Design review of the part built by this model. Coordinates are the model's own, in mm. Coordinates: 2 decimals unless noted, no trailing zeros. Write each loop counter-clockwise with the first axis right and the second up, starting at its lowest first coordinate (ties: lowest second). Pieces come first, ordered by that corner, then holes. Notation, with made-up numbers: (-35.5, 42.25) - (-25.5, 42.25) arc R29 ccw to (-25.5, 71.25) - close; hole circle Ø10 at (-17, 35.5). An arc over 180 degrees is marked (long way). One line per item, written item: value.
from build123d import *

# Parameters (mm, degrees)
CYLINDER021_R       = 5
CYLINDER021_DEPTH   = 15
CYLINDER107_R       = 1.6
CYLINDER107_DEPTH   = 20
ARRAY001008_X_COUNT = 2
ARRAY001008_X_PITCH = 22
ARRAY001008_Y_COUNT = 2
ARRAY001008_Y_PITCH = 22
BOX009_W            = 30
BOX009_H            = 30
BOX009_DEPTH        = 1
FILLET004_R         = 4


with BuildPart() as side_bearing_central_hole_cylinder001:
    # Cylinder021 → Cylinder021 (new body)
    with BuildSketch(Plane(origin=(15, 15, -4), x_dir=(1, 0, 0), z_dir=(0, 0, 1))):
        Circle(CYLINDER021_R)
    extrude(amount=CYLINDER021_DEPTH)


with BuildPart() as fusion010:
    # Cylinder107 → Cylinder107 (new body)
    with BuildSketch(Plane(origin=(4, 4, -7), x_dir=(1, 0, 0), z_dir=(0, 0, 1))):
        Circle(CYLINDER107_R)
    extrude(amount=CYLINDER107_DEPTH)

    # Array001008 X: Fusion010 ×2


with BuildPart() as fusion010_1:
    add(fusion010.part)
    with Locations(*[(i * ARRAY001008_X_PITCH, 0, 0) for i in range(1, ARRAY001008_X_COUNT)]):
        add(fusion010.part)

    # Array001008 Y: Fusion010 ×2


with BuildPart() as fusion010_2:
    add(fusion010_1.part)
    with Locations(*[(0, i * ARRAY001008_Y_PITCH, 0) for i in range(1, ARRAY001008_Y_COUNT)]):
        add(fusion010_1.part)

    # Fusion010: union side bearing central hole cylinder001
    add(side_bearing_central_hole_cylinder001.part)


with BuildPart() as bearing_cover_fillet:
    # Box009 → Box009 (new body)
    with BuildSketch(Plane.XY):
        with Locations((15, 15)):
            Rectangle(BOX009_W, BOX009_H)
    extrude(amount=BOX009_DEPTH)

    # Cut007: cut Fusion010
    add(fusion010_2.part, mode=Mode.SUBTRACT)

    # Fillet004
    fillet004_edges = [bearing_cover_fillet.edges().sort_by_distance(p)[0] for p in [
        (0, 0, 0.5),
        (0, 30, 0.5),
        (30, 0, 0.5),
        (30, 30, 0.5),
    ]]
    fillet(fillet004_edges, radius=FILLET004_R)


solid = bearing_cover_fillet.part
1. Consider section C-C, the plane y = 16.75. Write out the cut boundary in (x, z).
Answer block:
outline: (0, 0) - (10.32, 0) - (10.32, 1) - (0, 1) - close; (19.68, 0) - (30, 0) - (30, 1) - (19.68, 1) - close
2. Consider section A-A, the plane x = 27.25. Write out the cut boundary in (y, z), then the cut area to 3 significant figures.
Answer block:
outline: (0.2, 0) - (3, 0) - (3, 1) - (0.2, 1) - close; (5, 0) - (25, 0) - (25, 1) - (5, 1) - close; (27, 0) - (29.8, 0) - (29.8, 1) - (27, 1) - close
area: 25.6 mm^2
3. Wall thickness on line 1 along Y through (x, z) = (4, 0.35); line 2 along Y through (x, z) = (15, 0.45): over which ranges is each line inside the solid? List them lowest first.
Answer block:
line 1: y = 0 to 2.4, 5.6 to 24.4, 27.6 to 30
line 2: y = 0 to 10, 20 to 30
4. Consider section D-D, the plane x = 14.75. Write out the cut boundary in (y, z).
Answer block:
outline: (0, 0) - (10.01, 0) - (10.01, 1) - (0, 1) - close; (19.99, 0) - (30, 0) - (30, 1) - (19.99, 1) - close
5. Mouldability with a two-part tool opening along X and no side actions: class faces 1 (the face through (1.141, 28.797, 0.507)), 2 (the face through (28.797, 28.859, 0.507)), 3 (the face through (17.307, 10.564, 0.493)) as released by +X, released by -X, zero draft, split by the parting line, or undercut.
Answer block:
face 1: released by -X
face 2: released by +X
face 3: undercut
6. Consider section B-B, the plane z = 0.45. Write out the cut boundary in (x, y), then the cut area to 3 significant figures.
Answer block:
outline: (0, 4) arc R4 ccw to (4, 0) - (26, 0) arc R4 ccw to (30, 4) - (30, 26) arc R4 ccw to (26, 30) - (4, 30) arc R4 ccw to (0, 26) - close; hole circle Ø3.2 at (4, 4); hole circle Ø3.2 at (4, 26); hole circle Ø10 at (15, 15); hole circle Ø3.2 at (26, 4); hole circle Ø3.2 at (26, 26)
area: 776 mm^2
